Here's how the part is built. I have some questions about the finished solid (model axes, mm). Face numbers are marked on the shaded views. A direction names the side the tool comes from. Round coordinates to 2 decimals unless told otherwise and drop trailing zeros. Order: outer loops, then holes, each group sorted by start corner. A loop starts at its lowest first (then second) coordinate and runs counter-clockwise, first axis right, second up. Notation, with made-up numbers: (79.25, 81) -> (105.25, 81) arc R18 ccw to (105.25, 113) -> close; hole circle Ø4 at (86, 21.25). An arc over 180 degrees is marked (long way). Answer in a Markdown table with one row per item.
```python
from build123d import *

# Parameters (mm, degrees)
F0_R     = 11
F0_R_2   = 8.025
F0_R_3   = 6.025
F1_DEPTH = 26.05
F2_DEPTH = 16.78
F3_DEPTH = 13
F4_DEPTH = 7
F6_D     = 5.12
F6_DEPTH = 120
F6_TIP   = 1.5382031847


with BuildPart() as f1:
    # F0 (on Top) → F1 (new body)
    with BuildSketch(Plane.XY):
        Circle(F0_R)
        Circle(F0_R_2, mode=Mode.SUBTRACT)
        Circle(F0_R_2)
        Circle(F0_R_3, mode=Mode.SUBTRACT)
        Circle(F0_R_3)
    extrude(amount=-F1_DEPTH)

    # F0 (on Top) → F2 (join)
    with BuildSketch(Plane.XY):
        Circle(F0_R_2)
        Circle(F0_R_3, mode=Mode.SUBTRACT)
        Circle(F0_R_3)
    extrude(amount=F2_DEPTH)

    # F0 (on Top) → F3 (cut)
    with BuildSketch(Plane.XY):
        Circle(F0_R_2)
        Circle(F0_R_3, mode=Mode.SUBTRACT)
    extrude(amount=F3_DEPTH, mode=Mode.SUBTRACT)

    # F0 (on Top) → F4 (join)
    with BuildSketch(Plane.XY):
        Circle(F0_R_2)
        Circle(F0_R_3, mode=Mode.SUBTRACT)
    extrude(amount=F4_DEPTH)

    # F6
    with Locations(Plane(origin=(0, 0, -26.05), x_dir=(1, 0, 0), z_dir=(0, 0, -1))):
        with Locations((0, 0)):
            Hole(F6_D / 2, depth=F6_DEPTH)
            with Locations((0, 0, -(F6_DEPTH + F6_TIP / 2))):  # 118° drill point
                Cone(0, F6_D / 2, F6_TIP, mode=Mode.SUBTRACT)


solid = f1.part
```
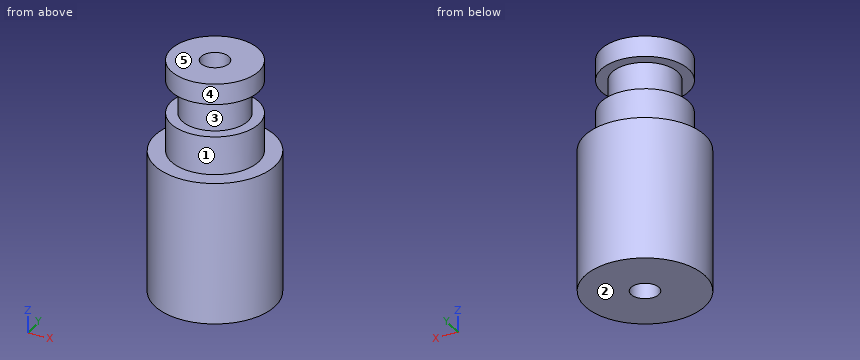
1. We'd pull the mould along Z, two halves only. Please class the marked faces 1, 2 and 3: released by +Z, released by -Z, zero draft, split by the parting line, or undercut.
Numbers:
| item | result |
|---|---|
| face 1 | zero draft |
| face 2 | released by -Z |
| face 3 | undercut |
2. For pin 1 Ø2 at (x, z) = (-3.5, -11.5) entering from -Y; pin 2 Ø10 at (x, z) = (-2, 9.5) entering from -Y (3 decimals); pin 3 Ø1 at (x, y) = (0.5, 0) entering from -Z; pin 4 Ø5 at (x, y) = (-1, -0.5) entering from +Z, each with a flat end and sliding along its axis, tell me the tip position at first contact or that it passes through.
Numbers:
| item | result |
|---|---|
| pin 1 | stops at y = -10.71 |
| pin 2 | stops at y = -8.025 |
| pin 3 | passes through |
| pin 4 | stops at z = 16.78 |
3. Suppose I cut it at C-C on z = 2. Write out the boundary of the cut face in (x, y) (3 decimals).
Numbers:
| item | result |
|---|---|
| outline | circle Ø16.05 at (0, 0); hole circle Ø5.12 at (0, 0) |
4. Suppose I cut it at A-A on x = 0. Write out the boundary of the cut face in (y, z) (3 decimals), then the cut area to 3 significant figures.
Numbers:
| item | result |
|---|---|
| outline | (-11, -26.05) -> (-2.56, -26.05) -> (-2.56, 16.78) -> (-8.025, 16.78) -> (-8.025, 13) -> (-6.025, 13) -> (-6.025, 7) -> (-8.025, 7) -> (-8.025, 0) -> (-11, 0) -> close; (2.56, -26.05) -> (11, -26.05) -> (11, 0) -> (8.025, 0) -> (8.025, 7) -> (6.025, 7) -> (6.025, 13) -> (8.025, 13) -> (8.025, 16.78) -> (2.56, 16.78) -> close |
| area | 599 mm2 |
5. Suppose I cut it at D-D on y = 3.75. Write out the boundary of the cut face in (x, z), then the cut area to 3 significant figures.
Numbers:
| item | result |
|---|---|
| outline | (-10.34, -26.05) -> (10.34, -26.05) -> (10.34, 0) -> (7.09, 0) -> (7.09, 7) -> (4.72, 7) -> (4.72, 13) -> (7.09, 13) -> (7.09, 16.78) -> (-7.09, 16.78) -> (-7.09, 13) -> (-4.72, 13) -> (-4.72, 7) -> (-7.09, 7) -> (-7.09, 0) -> (-10.34, 0) -> close |
| area | 748 mm2 |
6. For the marked faces 4 and 5, which set-ups out of +Z, -Z, +X, -X, +Y, -Y let a thin tool reach every point of the face, with its end or its side?
Numbers:
| item | result |
|---|---|
| face 4 | +Z |
| face 5 | +Z, +X, -X, +Y, -Y |
7. Please list where these lines run through material, in increasing order: line 1 along Z through (x, y) = (1.5, 7.5); line 2 along Y through (x, z) = (0, 4.5) (3 decimals); line 3 along Y through (x, z) = (0, -15).
Numbers:
| item | result |
|---|---|
| line 1 | z = -26.05 to 7, 13 to 16.78 |
| line 2 | y = -8.025 to -2.56, 2.56 to 8.025 |
| line 3 | y = -11 to -2.56, 2.56 to 11 |
